Autodesk Inventor part; units mm, degrees
ref_plane "YZ Plane" through (0, 0, 0) normal (1, 0, 0) x (0, 1, 0)
ref_plane "XZ Plane" through (0, 0, 0) normal (0, 1, 0) x (-1, 0, 0)
ref_plane "XY Plane" through (0, 0, 0) normal (0, 0, 1) x (1, 0, 0)
sketch "Эскиз1" plane through (0, 0, 0) normal (0, 0, 1) x (1, 0, 0)
  arc A0 (0.9499, 0.3125) -> (0.1, 0.995) centre (0, 0) ccw
  line L0 (0.9499, 0.3125) -> (1.4499, 0.3125)
  line L1 (1.4499, 0.3125) -> (1.4499, -0.1875)
  line L2 (1.4499, -0.1875) -> (0.9823, -0.1875)
  arc A1 (0.1, -0.995) -> (0.9823, -0.1875) centre (0, 0) ccw
  line L3 (0.1, -0.995) -> (0.1, -4.5)
  line L4 (0.1, -4.5) -> (0.3, -4.7)
  line L5 (0.3, -4.7) -> (8.9, -4.7)
  line L6 (8.9, -4.7) -> (9.1, -4.5)
  line L7 (9.1, -4.5) -> (9.1, -0.995)
  arc A2 (8.2177, -0.1875) -> (9.1, -0.995) centre (9.2, 0) ccw
  line L8 (8.2177, -0.1875) -> (7.7501, -0.1875)
  line L9 (7.7501, -0.1875) -> (7.7501, 0.3125)
  line L10 (7.7501, 0.3125) -> (8.2501, 0.3125)
  arc A3 (9.1, 0.995) -> (8.2501, 0.3125) centre (9.2, 0) ccw
  line L11 (9.1, 0.995) -> (9.1, 1.6)
  line L12 (9.1, 1.6) -> (8.9, 1.8)
  line L13 (8.9, 1.8) -> (0.3, 1.8)
  line L14 (0.3, 1.8) -> (0.1, 1.6)
  line L15 (0.1, 1.6) -> (0.1, 0.995)
extrude "Выдавливание1" add sketch "Эскиз1" along normal blind 220
sketch "Эскиз2" plane through (0.3, 1.8, 0) normal (0, 1, 0) x (1, 0, 0)
  line L0 (4.3, 0) -> (4.3, -40) construction
  circle A0 centre (4.3, -7.5) radius 3
  line L1 (8.6, 0) -> (0, 0)
  dimension "d3" = 6
  dimension "d25" = 7.5
extrude "Выдавливание2" cut sketch "Эскиз2" against normal blind 3.5
sketch "Эскиз3" plane through (0.3, -4.7, 0) normal (0, -1, 0) x (1, 0, 0)
  line L0 (0, 0) -> (8.6, 0) construction
  line L1 (4.3, 0) -> (4.3, 8.2468) construction
  circle A0 centre (4.3, 7.5) radius 1.75
  point P0 (-0.3, 0)
  dimension "d26" = 3.5
  dimension "d27" = 7.5
extrude "Выдавливание3" cut sketch "Эскиз3" against normal blind 5
chamfer "Фаска1" distance 0.2 angle 45 2 edges at (2.85, -4.7, 7.5) (1.6, 1.8, 7.5)
pattern_linear "Прямоуг.массив1" count 11 spacing 20 along (0, 0, 1) of "Выдавливание3", "Выдавливание2", "Фаска1"
properties part number "рельса_центр"
Check sheet for the modelled part. Datum: model origin and axes. Units: mm. A direction names the side the tool comes from. Give positions to 0.01 mm unless a question says otherwise; leave off trailing zeros. One line per item, written item: value. Start each with the question number.
Item 1: Material ranges on probe 1 along X at (y, z) = (-2.75, 167.5); probe 2 along Y at (x, z) = (1.25, 85.5); probe 3 along X at (y, z) = (0.55, 147.5), recorded low to high. Write a range as from..to.
Item 2: Draft check along X on faces 3 (the flat face through (6, -1.7, 169)), 4 (the flat face through (5, -1, 220)), 5 (the flat face through (9.1, -3, 108)). Enter one of: +X half, -X half, draft (parallel to the pull), parting line (faces both ways), or undercut.
Item 3: Tool access check on faces 1 (the cylindrical face through (4.372, -3.12, 29.235)), 2 (the flat face through (6, -1.7, 49)). Record the directions out of +Z, -Z, +X, -X, +Y, -Y that give a thin tool (end or side, any length) a straight path to the whole face; none if there is none.
Item 4: Gauge pin test, flat ends, axial feed: pin 1 (4 mm diameter, centred on x = 4.6, z = 127.5, fed in from +Y); pin 2 (1 mm diameter, centred on x = 5, y = -4, fed in from -Z). Record the tip position at first contact, or that the pin passes through.
Item 5: Section check B-B on y = -3.5. State how many separate pieces and enclosed holes the cut face has, then the cut area to 3 significant figures.
Results list:
1. probe 1: 0.1..2.85, 6.35..9.1
1. probe 2: -4.7..-0.19, 0.31..1.8
1. probe 3: 0.84..1.6, 7.6..8.36
2. face 3: undercut
2. face 4: draft
2. face 5: +X half
3. face 1: +Y, -Y
3. face 2: +Y
4. pin 1: y = -1.7
4. pin 2: z = 0
5. separate pieces: 1
5. enclosed holes: 11
5. area: 1,870 mm²
